Design review of the part built by this model. Coordinates are the model's own, in mm. A direction names the side the tool comes from. Round coordinates to 2 decimals unless told otherwise and drop trailing zeros. Order: outer loops, then holes, each group sorted by start corner. A loop starts at its lowest first (then second) coordinate and runs counter-clockwise, first axis right, second up. Notation, with made-up numbers: M -20,-8 L 25,-8 A25 ccw 25,13 Z; hole C 52,-29.5 d2. An arc over 180 degrees is marked long. Write item = value, one per line. Start each with the question number.
```python
from build123d import *

# Parameters (mm, degrees)
F0_W     = 60
F0_H     = 60
F1_DEPTH = 1
F4_DEPTH = 1
F5_DEPTH = 29
F6_W     = 1
F6_H     = 1


with BuildPart() as f1:
    # F0 (on Top) → F1 (new body)
    with BuildSketch(Plane.XY):
        Rectangle(F0_W, F0_H)
    extrude(amount=F1_DEPTH)

    # F3 (on face) → F4 (cut, through all)
    with BuildSketch(Plane.XY.offset(1)):
        Polygon((-30, -30), (16, -30), (-30, 3.8595641273), align=None)
    extrude(amount=-F4_DEPTH, mode=Mode.SUBTRACT)

    # F2 (on Right) → F5 (cut, symmetric)
    with BuildSketch(Plane.YZ):
        Polygon((11.2525225805, 0), (17, 0), (17, 1), (14, 1), align=None)
    extrude(amount=F5_DEPTH, both=True, mode=Mode.SUBTRACT)

    # F6 (on face) → F7 (join, up to the next surface of F1)
    with BuildSketch(Plane.XZ.offset(-17)):
        with Locations((-22.125, 0.5)):
            Rectangle(F6_W, F6_H)
        with Locations((-14.75, 0.5)):
            Rectangle(F6_W, F6_H)
        with Locations((-7.375, 0.5)):
            Rectangle(F6_W, F6_H)
        with Locations((0, 0.5)):
            Rectangle(F6_W, F6_H)
        with Locations((7.375, 0.5)):
            Rectangle(F6_W, F6_H)
        with Locations((14.75, 0.5)):
            Rectangle(F6_W, F6_H)
        with Locations((22.125, 0.5)):
            Rectangle(F6_W, F6_H)
    extrude(until=Until.NEXT)


solid = f1.part
```
(1) Consider section A-A, the plane x = 26. Write out the cut boundary in (y, z).
(2) Consider section C-C, the plane x = 2.5. Write out the cut boundary in (y, z), then the cut area to 3 significant figures.
(3) Consider section B-B, the plane y = 15. State how many separate pieces and enclosed holes the cut face has, then the cut area to 3 significant figures.
(4) Draft analysis for pull direction Y (two halves, no side actions). For faces 1 (the face through (6, 7, 1)), 2 (the face through (-3.64, 12.65, 0.51)), 3 (the face through (-6.678, -13.307, 0.507)), state which applies: pulls with the +Y half, pulls with the -Y half, needs draft (parallel to the pull), parting line crosses it, or undercut.
(5) Insertion check: pin 1 (0.5 mm diameter, centred on x = 3.5, z = 0.5, fed in from -Y); pin 2 (0.5 mm diameter, centred on x = -10.5, z = 0.5, fed in from -Y); pin 3 (0.5 mm diameter, centred on x = -4, z = 0.5, fed in from -Y). Each pin has a flat end and moves straight along its axis. Give the tip position at first contact, or say it passes through.
(6) For faces 4 (the face through (-11.02, 12.65, 0.51)), 5 (the face through (6, 7, 0)), list the 3-axis set-ups (+Z, -Z, +X, -X, +Y, -Y) from which the entire face can be reached by the end or side of a thin tool; tool diameter is ignored.
(7) For line 1 along X through (y, z) = (-1, 0.9); line 2 along Y through (x, z) = (14.5, 0.1); line 3 along Y through (x, z) = (-22.5, 0.35), list the stretches that pass through material, from the lowest coordinate up. Write a range as [from, to].
Completed:
q1.outline = M -30,0 L 11.25,0 L 14,1 L -30,1 Z; M 17,0 L 30,0 L 30,1 L 17,1 Z
q2.outline = M -20.06,0 L 11.25,0 L 14,1 L -20.06,1 Z; M 17,0 L 30,0 L 30,1 L 17,1 Z
q2.area = 45.7 mm2
q3.separate_pieces = 9
q3.enclosed_holes = 0
q3.area = 9.00 mm2
q4.face_1 = needs draft
q4.face_2 = undercut
q4.face_3 = pulls with the -Y half
q5.pin_1 = -20.98
q5.pin_2 = -10.68
q5.pin_3 = -15.46
q6.face_4 = -Z
q6.face_5 = -Z, +X, -X, +Y, -Y
q7.line_1 = [-23.4, 30]
q7.line_2 = [-28.9, 30]
q7.line_3 = [-1.66, 30]
